```python
from build123d import *

# Parameters (mm, degrees)
BOSS_EXTRUDE1_DEPTH      = 12.5
SKETCH2_R                = 0.75
CUT_EXTRUDE1_DEPTH       = 4
BOSS_EXTRUDE2_DEPTH      = 4
BOSS_EXTRUDE2_DEPTH_BACK = 4
SKETCH3_R                = 0.5
BOSS_EXTRUDE3_DEPTH      = 4
BOSS_EXTRUDE3_DEPTH_BACK = 4
SKETCH4_R                = 0.5


with BuildPart() as part:
    # Sketch1 → Boss-Extrude1 (new body)
    with BuildSketch(Plane(origin=(0, 0, 0), x_dir=(1, 0, 0), z_dir=(0, 1, 0))):
        with BuildLine():
            Line((-1.578824879, 1.227726355), (1.578824879, 1.227726355))
            ThreePointArc((1.578824879, 1.227726355), (2, 0), (1.578824879, -1.227726355))
            Line((1.578824879, -1.227726355), (-1.578824879, -1.227726355))
            ThreePointArc((-1.578824879, -1.227726355), (-2, 0), (-1.578824879, 1.227726355))
        make_face()
    extrude(amount=BOSS_EXTRUDE1_DEPTH)

    # Sketch2 → Cut-Extrude1 (cut)
    with BuildSketch(Plane(origin=(0, 12.5, 0), x_dir=(1, 0, 0), z_dir=(0, 1, 0))):
        with Locations(Location((0, 0, 0), (0, 0, 270))):
            Circle(SKETCH2_R)
    extrude(amount=-CUT_EXTRUDE1_DEPTH, mode=Mode.SUBTRACT)

    # Sketch3 → Boss-Extrude2 (add, two sides: drawn at the far end of the back side and taken through both)
    with BuildSketch(Plane.XY.offset(-BOSS_EXTRUDE2_DEPTH_BACK)):
        Circle(SKETCH3_R)
    extrude(amount=BOSS_EXTRUDE2_DEPTH + BOSS_EXTRUDE2_DEPTH_BACK)

    # Sketch4 → Boss-Extrude3 (add, two sides: drawn at the far end of the back side and taken through both)
    with BuildSketch(Plane(origin=(0, 0, 0), x_dir=(0, 0, -1), z_dir=(1, 0, 0)).offset(-BOSS_EXTRUDE3_DEPTH_BACK)):
        Circle(SKETCH4_R)
    extrude(amount=BOSS_EXTRUDE3_DEPTH + BOSS_EXTRUDE3_DEPTH_BACK)


solid = part.part
```
Check sheet for the modelled part. Datum: model origin and axes. Units: mm. A direction names the side the tool comes from. Coordinates: 2 decimals unless noted, no trailing zeros. Loops run counter-clockwise (first coordinate to the right, second up) from the corner with the lowest first, then second, coordinate; pieces in that order, holes last. Notation, with made-up numbers: M 50,32.25 L 93,32.25 A16 ccw 93,56.25 Z; hole C 2,-37 d1. An arc over 180 degrees is marked long. Answer as a JSON object with one key per item and string values.
1. Sectioned sample at C-C on y = 6.75. Record the cut outline in (x, z), and give its area (3 significant figures).
Outcome:
{"outline": "M -1.58,-1.23 L 1.58,-1.23 A2 ccw 1.58,1.23 L -1.58,1.23 A2 ccw Z", "area": "9.16 mm²"}
2. Access from +Z, -Z, +X, -X, +Y, -Y to the whole of each face (thin tool, end or side, straight path). Record for faces 5 (the cylindrical face through (-0.108, -0.488, -2.472)), 6 (the cylindrical face through (2.416, -0.488, 0.108)), 7 (the cylindrical face through (-0.108, -0.488, 2.416)), 8 (the cylindrical face through (-2.472, -0.488, 0.108)), 9 (the cylindrical face through (-2, 6, 0)).
Outcome:
{"face 5": "-Z", "face 6": "+X", "face 7": "+Z", "face 8": "-X", "face 9": "-X, +Y"}
3. Depth check by flat-ended pin: P1, Ø0.8, axis at x = -1, z = -0.5, coming from the -Y side; P2, Ø3, axis at y = 6.5, z = 1, coming from the -X side; P3, Ø0.8, axis at x = 1.5, z = 1, coming from the -Y side. Enter the tip coordinate at first touch or a pass-through.
Outcome:
{"P1": "y = -0.49", "P2": "x = -2", "P3": "y = 0"}
4. Sectioned sample at B-B on z = 3.75. Record the cut outline in (x, y), and give its area (3 significant figures).
Outcome:
{"outline": "C 0,0 d1", "area": "0.785 mm²"}
5. Scan lines: L1, parallel to X at y = 10.3, z = 0; L2, parallel to Y at x = 0, z = -2.5; L3, parallel to Z at x = -0.5, y = 9.25. Record each from-to range of solid material in increasing order. Write a range as from..to.
Outcome:
{"L1": "-2..-0.75, 0.75..2", "L2": "-0.5..0.5", "L3": "-1.23..-0.56, 0.56..1.23"}
6. Release check for a two-part mould opening along Z. For faces 1 (the flat face through (-4, 0, 0)), 2 (the flat face through (0, 8.5, 0)), 3 (the flat face through (0, 6, -1.228)), 4 (the cylindrical face through (0.225, 10.528, 0.715)) record: pulls with the +Z half, pulls with the -Z half, needs draft (parallel to the pull), parting line crosses it, or undercut.
Outcome:
{"face 1": "needs draft", "face 2": "undercut", "face 3": "pulls with the -Z half", "face 4": "undercut"}
7. Sectioned sample at A-A on x = 1.25. Record the cut outline in (y, z).
Outcome:
{"outline": "M 0,-1.23 L 12.5,-1.23 L 12.5,1.23 L 0,1.23 L 0,0.5 A0.5 ccw 0,-0.5 Z"}
